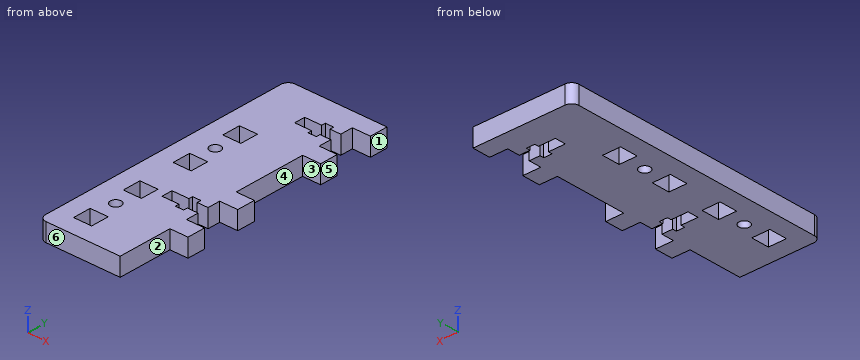
from build123d import *

# Parameters (mm, degrees)
SKETCH1_W           = 5
SKETCH1_H           = 5
SKETCH1_R           = 1.5
BOSS_EXTRUDE1_DEPTH = 5
CONG_1_R            = 2


with BuildPart() as part:
    # Sketch1 → Boss-Extrude1 (new body)
    with BuildSketch(Plane.XY):
        Polygon((22.5, 35), (22.5, 55), (27.5, 55), (27.5, 60), (22.5, 60), (22.5, 63.5), (19.5, 63.5), (19.5, 62.4), (17.2, 62.4), (17.2, 63.5), (12.5, 63.5), (12.5, 66.5), (17.2, 66.5), (17.2, 67.6), (19.5, 67.6), (19.5, 66.5), (22.5, 66.5), (22.5, 70), (27.5, 70), (27.5, 75), (22.5, 75), (0, 75), (0, 0), (22.5, 0), (22.5, 15), (27.5, 15), (27.5, 20), (22.5, 20), (22.5, 23.5), (19.5, 23.5), (19.5, 22.4), (17.2, 22.4), (17.2, 23.5), (12.5, 23.5), (12.5, 26.5), (17.2, 26.5), (17.2, 27.6), (19.5, 27.6), (19.5, 26.5), (22.5, 26.5), (22.5, 30), (27.5, 30), (27.5, 35), align=None)
        with Locations((7.5, 7.5)):
            Rectangle(SKETCH1_W, SKETCH1_H, mode=Mode.SUBTRACT)
        with Locations((7.5, 15)):
            Circle(SKETCH1_R, mode=Mode.SUBTRACT)
        with Locations((7.5, 22.5)):
            Rectangle(SKETCH1_W, SKETCH1_H, mode=Mode.SUBTRACT)
        with Locations((7.5, 37.5)):
            Rectangle(SKETCH1_W, SKETCH1_H, mode=Mode.SUBTRACT)
        with Locations((7.5, 45)):
            Circle(SKETCH1_R, mode=Mode.SUBTRACT)
        with Locations((7.5, 52.5)):
            Rectangle(SKETCH1_W, SKETCH1_H, mode=Mode.SUBTRACT)
    extrude(amount=BOSS_EXTRUDE1_DEPTH)

    # Congé1
    cong_1_edges = [part.edges().sort_by_distance(p)[0] for p in [
        (0, 0, 2.5),
        (0, 75, 2.5),
    ]]
    fillet(cong_1_edges, radius=CONG_1_R)


solid = part.part
Design review of the part built by this model. Coordinates are the model's own, in mm. Face numbers are marked on the shaded views. A direction names the side the tool comes from. Give positions to 0.01 mm unless a question says otherwise; leave off trailing zeros. Loops run counter-clockwise (first coordinate to the right, second up) from the corner with the lowest first, then second, coordinate; pieces in that order, holes last. Notation, with made-up numbers: M -15.75,-36 L 22.25,-36 A22 ccw 22.25,-22 Z; hole C 40.25,46.5 d11. An arc over 180 degrees is marked long. One line per question, with ' | ' between items. Start each with the question number.
1. Add section B-B (x = 24). Write out the cut boundary in (y, z), plus the area to 3 significant figures.
2. For the marked faces 1, 2 and 3, list the 3-axis set-ups (+Z, -Z, +X, -X, +Y, -Y) from which the entire face can be reached by the end or side of a thin tool; tool diameter is ignored.
3. Add section C-C (y = 45). Write out the cut boundary in (x, z), plus the area to 3 significant figures.
4. To check wall thickness, follow L1, parallel to Y at x = 20.5, z = 4.2; L2, parallel to Y at x = 25.75, z = 3.55; L3, parallel to Y at x = 5.5, z = 1.15. State the ranges of each line that lie inside material, in increasing order.
5. Add section A-A (x = 7.5). Write out the cut boundary in (y, z), plus the area to 3 significant figures.
6. Insertion check: P1, Ø2.5, axis at y = 22.5, z = 3.5, coming from the +X side; P2, Ø3, axis at x = 19, y = 60.5, coming from the -Z side. Each pin has a flat end and moves straight along its axis. Give the tip position at first contact, or say it passes through.
7. Add section D-D (y = 37). Write out the cut boundary in (x, z).
8. The part is to be moulded in two halves that separate along Y. For the marked faces 4, 5 and 6, say which applies: released by +Y, released by -Y, zero draft, split by the parting line, or undercut.
Worked out:
1) outline: M 15,0 L 20,0 L 20,5 L 15,5 Z; M 30,0 L 35,0 L 35,5 L 30,5 Z; M 55,0 L 60,0 L 60,5 L 55,5 Z; M 70,0 L 75,0 L 75,5 L 70,5 Z | area: 100 mm²
2) face 1: +Z, -Z, +X, +Y, -Y | face 2: +Z, -Z, +X, -Y | face 3: +Z, -Z, +X
3) outline: M 0,0 L 6,0 L 6,5 L 0,5 Z; M 9,0 L 22.5,0 L 22.5,5 L 9,5 Z | area: 97.5 mm²
4) L1: y = 0 to 23.5, 26.5 to 63.5, 66.5 to 75 | L2: y = 15 to 20, 30 to 35, 55 to 60, 70 to 75 | L3: y = 0 to 5, 10 to 20, 25 to 35, 40 to 50, 55 to 75
5) outline: M 0,0 L 5,0 L 5,5 L 0,5 Z; M 10,0 L 13.5,0 L 13.5,5 L 10,5 Z; M 16.5,0 L 20,0 L 20,5 L 16.5,5 Z; M 25,0 L 35,0 L 35,5 L 25,5 Z; M 40,0 L 43.5,0 L 43.5,5 L 40,5 Z; M 46.5,0 L 50,0 L 50,5 L 46.5,5 Z; M 55,0 L 75,0 L 75,5 L 55,5 Z | area: 245 mm²
6) P1: stops at x = 22.5 | P2: stops at z = 0
7) outline: M 0,0 L 5,0 L 5,5 L 0,5 Z; M 10,0 L 22.5,0 L 22.5,5 L 10,5 Z
8) face 4: undercut | face 5: zero draft | face 6: released by -Y
